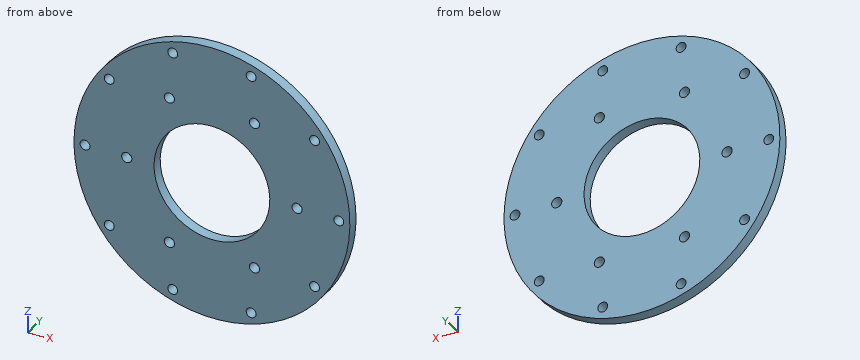
from build123d import *

# Parameters (mm, degrees)
SKETCH2_R           = 40.5
SKETCH2_R_2         = 17
SKETCH2_R_3         = 1.45
SKETCH2_R_4         = 1.5
BOSS_EXTRUDE1_DEPTH = 3.175


with BuildPart() as part:
    # Sketch2 → Boss-Extrude1 (new body)
    with BuildSketch(Plane(origin=(0, 0, 0), x_dir=(1, 0, 0), z_dir=(0, 1, 0))):
        with Locations(Location((0, 0, 0), (0, 0, 270))):
            Circle(SKETCH2_R)
        with Locations(Location((0, 0, 0), (0, 0, 270))):
            Circle(SKETCH2_R_2, mode=Mode.SUBTRACT)
        with Locations(Location((-37.25, 0, 0), (0, 0, 270))):
            Circle(SKETCH2_R_3, mode=Mode.SUBTRACT)
        with Locations(Location((-25, 0, 0), (0, 0, 270))):
            Circle(SKETCH2_R_4, mode=Mode.SUBTRACT)
        with Locations(Location((-12.5, 21.650635095, 0), (0, 0, 270))):
            Circle(SKETCH2_R_4, mode=Mode.SUBTRACT)
        with Locations(Location((12.5, 21.650635095, 0), (0, 0, 270))):
            Circle(SKETCH2_R_4, mode=Mode.SUBTRACT)
        with Locations(Location((25, 0, 0), (0, 0, 270))):
            Circle(SKETCH2_R_4, mode=Mode.SUBTRACT)
        with Locations(Location((12.5, -21.650635095, 0), (0, 0, 270))):
            Circle(SKETCH2_R_4, mode=Mode.SUBTRACT)
        with Locations(Location((-12.5, -21.650635095, 0), (0, 0, 270))):
            Circle(SKETCH2_R_4, mode=Mode.SUBTRACT)
        with Locations(Location((-30.13588304, 21.895000648, 0), (0, 0, 270))):
            Circle(SKETCH2_R_3, mode=Mode.SUBTRACT)
        with Locations(Location((-11.51088304, 35.426855232, 0), (0, 0, 270))):
            Circle(SKETCH2_R_3, mode=Mode.SUBTRACT)
        with Locations(Location((11.51088304, 35.426855232, 0), (0, 0, 270))):
            Circle(SKETCH2_R_3, mode=Mode.SUBTRACT)
        with Locations(Location((30.13588304, 21.895000648, 0), (0, 0, 270))):
            Circle(SKETCH2_R_3, mode=Mode.SUBTRACT)
        with Locations(Location((37.25, 0, 0), (0, 0, 270))):
            Circle(SKETCH2_R_3, mode=Mode.SUBTRACT)
        with Locations(Location((30.13588304, -21.895000648, 0), (0, 0, 270))):
            Circle(SKETCH2_R_3, mode=Mode.SUBTRACT)
        with Locations(Location((11.51088304, -35.426855232, 0), (0, 0, 270))):
            Circle(SKETCH2_R_3, mode=Mode.SUBTRACT)
        with Locations(Location((-11.51088304, -35.426855232, 0), (0, 0, 270))):
            Circle(SKETCH2_R_3, mode=Mode.SUBTRACT)
        with Locations(Location((-30.13588304, -21.895000648, 0), (0, 0, 270))):
            Circle(SKETCH2_R_3, mode=Mode.SUBTRACT)
    extrude(amount=BOSS_EXTRUDE1_DEPTH)


solid = part.part
Geometry: final body of the model. Coordinates: model frame, mm. Coordinates: 2 decimals unless noted, no trailing zeros. Order: outer loops, then holes, each group sorted by start corner. A loop starts at its lowest first (then second) coordinate and runs counter-clockwise, first axis right, second up. Notation, with made-up numbers: (26, -11.5) - (55, -11.5) arc R20 ccw to (55, -2.5) - close; hole circle Ø2 at (-32.5, 18). An arc over 180 degrees is marked (long way). Use one line per item in the form item = value.
1) Section C-C (y = 1.3). State how many separate pieces and enclosed holes the cut face has, then the cut area to 3 significant figures.
Solutions:
separate_pieces = 1
enclosed_holes = 17
area = 4,140 mm^2
2) Section A-A (z = 0). Return loops of the section in (x, y) (3 decimals), then the cut area to 3 significant figures.
Solutions:
outline = (-40.5, 0) - (-38.7, 0) - (-38.7, 3.175) - (-40.5, 3.175) - close; (-35.8, 0) - (-26.5, 0) - (-26.5, 3.175) - (-35.8, 3.175) - close; (-23.5, 0) - (-17, 0) - (-17, 3.175) - (-23.5, 3.175) - close; (17, 0) - (23.5, 0) - (23.5, 3.175) - (17, 3.175) - close; (26.5, 0) - (35.8, 0) - (35.8, 3.175) - (26.5, 3.175) - close; (38.7, 0) - (40.5, 0) - (40.5, 3.175) - (38.7, 3.175) - close
area = 112 mm^2
3) Section B-B (x = -25). Return loops of the section in (y, z) (3 decimals), then the cut area to 3 significant figures.
Solutions:
outline = (0, -31.863) - (3.175, -31.863) - (3.175, -1.5) - (0, -1.5) - close; (0, 1.5) - (3.175, 1.5) - (3.175, 31.863) - (0, 31.863) - close
area = 193 mm^2
4) Ray query, L1, parallel to X at y = 1.85, z = 0; L2, parallel to X at y = 1.2, z = 35.5; L3, parallel to Z at x = 13.5, y = 1.4. Return the intervals inside material, ascending.
Solutions:
L1 = -40.5 to -38.7, -35.8 to -26.5, -23.5 to -17, 17 to 23.5, 26.5 to 35.8, 38.7 to 40.5
L2 = -19.49 to -12.96, -10.06 to 10.06, 12.96 to 19.49
L3 = -38.18 to -22.77, -20.53 to -10.33, 10.33 to 20.53, 22.77 to 38.18
5) Section D-D (x = -6). Return loops of the section in (y, z) (3 decimals).
Solutions:
outline = (0, -40.053) - (3.175, -40.053) - (3.175, -15.906) - (0, -15.906) - close; (0, 15.906) - (3.175, 15.906) - (3.175, 40.053) - (0, 40.053) - close
6) Pin query (flat end, axial travel): pin 1 (1.5 mm diameter, centred on x = 29, y = 2.5, fed in from -Z); pin 2 (1.5 mm diameter, centred on x = -27.5, y = 1.5, fed in from -Z). Return the tip coordinate at first contact, or that it passes through.
Solutions:
pin_1 = -29.02
pin_2 = -30.41
